from build123d import *

# Parameters (mm, degrees)
F0_R     = 60
F1_DEPTH = 20
F2_R     = 35
F3_DEPTH = 100
F5_DEPTH = 100


with BuildPart() as f1:
    # F0 (on Top) → F1 (new body)
    with BuildSketch(Plane.XY):
        Circle(F0_R)
    extrude(amount=F1_DEPTH)

    # F2 (on face) → F3 (join)
    with BuildSketch(Plane(origin=(0, 0, 0), x_dir=(1, 0, 0), z_dir=(0, 0, -1))):
        Circle(F2_R)
    extrude(amount=F3_DEPTH)

    # F4 (on face) → F5 (cut)
    with BuildSketch(Plane(origin=(0, 0, -100), x_dir=(1, 0, 0), z_dir=(0, 0, -1))):
        with BuildLine():
            Line((-7.8536700457, -25.464490056), (-7.8536700457, -28.953753933))
            ThreePointArc((-7.8536700457, -28.953753933), (2.2773518168, -29.913436257), (12.1463299543, -27.4311259091))
            Line((12.1463299543, -27.4311259091), (12.1463299543, -25.464490056))
            Line((12.1463299543, -25.464490056), (-7.8536700457, -25.464490056))
        make_face()
        with BuildLine():
            ThreePointArc((12.1463299543, -27.4311259091), (25.1434872147, -16.3647502482), (30, 0))
            ThreePointArc((30, 0), (-18.22621599, 23.8286602789), (-7.8536700457, -28.953753933))
            Line((-7.8536700457, -28.953753933), (-7.8536700457, -25.464490056))
            Line((-7.8536700457, -25.464490056), (12.1463299543, -25.464490056))
            Line((12.1463299543, -25.464490056), (12.1463299543, -27.4311259091))
        make_face()
        with BuildLine():
            ThreePointArc((12.1463299543, -27.4311259091), (2.2773518168, -29.913436257), (-7.8536700457, -28.953753933))
            Line((-7.8536700457, -28.953753933), (-7.8536700457, -34.1074752336))
            ThreePointArc((-7.8536700457, -34.1074752336), (2.2401014005, -34.9282399459), (12.1463299543, -32.824787412))
            Line((12.1463299543, -32.824787412), (12.1463299543, -27.4311259091))
        make_face()
    extrude(amount=-F5_DEPTH, mode=Mode.SUBTRACT)


solid = f1.part
Verification items for the finished model (mm, model axes). A direction names the side the tool comes from. Give positions to 0.01 mm unless a question says otherwise; leave off trailing zeros. Write each loop counter-clockwise with the first axis right and the second up, starting at its lowest first coordinate (ties: lowest second). Pieces come first, ordered by that corner, then holes. Notation, with made-up numbers: M -21.5,-3.75 L 9.5,-3.75 A30 cw 9.5,32.25 Z; hole C -1,53.5 d7. An arc over 180 degrees is marked long. Write item = value, one per line.
(1) Sectioned sample at B-B (z = -56.5). Record the cut outline in (x, y), then the cut area to 3 significant figures.
Found:
outline = M -7.85,28.95 L -7.85,34.11 A35 ccw long 12.15,32.82 L 12.15,27.43 A30 cw long Z
area = 919 mm2
(2) Sectioned sample at C-C (y = -5.5). Record the cut outline in (x, z), then the cut area to 3 significant figures.
Found:
outline = M -59.75,0 L -34.57,0 L -34.57,-100 L -29.49,-100 L -29.49,0 L 29.49,0 L 29.49,-100 L 34.57,-100 L 34.57,0 L 59.75,0 L 59.75,20 L -59.75,20 Z
area = 3,400 mm2
(3) Sectioned sample at D-D (x = 28). Record the cut outline in (y, z), then the cut area to 3 significant figures.
Found:
outline = M -53.07,0 L -21,0 L -21,-100 L -10.77,-100 L -10.77,0 L 10.77,0 L 10.77,-100 L 21,-100 L 21,0 L 53.07,0 L 53.07,20 L -53.07,20 Z
area = 4,170 mm2
(4) Material ranges on line 1 (X direction, y = 1, z = -49); line 2 (Z direction, x = 41, y = -5); line 3 (Y direction, x = 0, z = -73), recorded low to high.
Found:
line_1 = -34.99 to -29.98, 29.98 to 34.99
line_2 = 0 to 20
line_3 = -35 to -30
(5) Access from +Z, -Z, +X, -X, +Y, -Y to the whole of each face (thin tool, end or side, straight path). Record for faces 4 (the face through (-0.84, -34.99, -49.3)), 5 (the face through (-7.854, 31, -51)).
Found:
face_4 = -Z
face_5 = -Z, +Y
(6) Sectioned sample at A-A (x = 0). Record the cut outline in (y, z).
Found:
outline = M -60,0 L -35,0 L -35,-100 L -30,-100 L -30,0 L 60,0 L 60,20 L -60,20 Z
(7) Draft check along Z on faces 1 (the face through (-1, 1, 20)), 2 (the face through (10, -29, -100)), 3 (the face through (-59.94, 2.64, 9.86)). Enter one of: released by +Z, released by -Z, zero draft, split by the parting line, or undercut.
Found:
face_1 = released by +Z
face_2 = released by -Z
face_3 = zero draft
(8) Go/stop test with flat-tipped pins: pin 1 Ø4.5 at (y, z) = (31, -39.5) entering from -X; pin 2 Ø10 at (x, z) = (48, -2) entering from -Y; pin 3 Ø3 at (x, z) = (0.5, -4.5) entering from -Y. Record where each tip stops, or that it passes through.
Found:
pin_1 = -19.96
pin_2 = -41.41
pin_3 = -35
